Geometry: final body of the model. Coordinates: model frame, mm. A direction names the side the tool comes from. Round coordinates to 2 decimals unless told otherwise and drop trailing zeros. Loops run counter-clockwise (first coordinate to the right, second up) from the corner with the lowest first, then second, coordinate; pieces in that order, holes last. Notation, with made-up numbers: (10.5, 9.25) - (46.5, 9.25) arc R31 ccw to (46.5, 39.25) - close; hole circle Ø4 at (-21.75, 4.5). An arc over 180 degrees is marked (long way). Answer as a JSON object with one key per item and string values. Group by question number.
Item 1: Section D-D (z = 42.5). Return the cut outline in (x, y), plus the area to 3 significant figures.
Item 2: First-contact query: pin 1 (2 mm diameter, centred on y = 15, z = 30.5, fed in from -X); pin 2 (4 mm diameter, centred on x = 44.5, z = -7, fed in from +Y); pin 3 (4 mm diameter, centred on x = 51.16, z = 29.39, fed in from -Y). Flat tips, straight axial feed; report the tip coordinate or a pass-through.
Item 3: Section C-C (x = 40). Return the cut outline in (y, z), plus the area to 3 significant figures.
Item 4: Section B-B (y = 14). Return the cut outline in (x, z).
Item 5: Reachability of faces 4 (the face through (-49.787, 24.294, -11.056)), 5 (the face through (-56, 41, 0)), 6 (the face through (50.249, 43.028, 28.195)) from +Z, -Z, +X, -X, +Y, -Y: full face, straight path, thin tool, end or side. Return the list, or none.
Item 6: Section A-A (z = 0). Return the cut outline in (x, y).
Item 7: Line query: line 1 (Z direction, x = 1.5, y = 22.5); line 2 (X direction, y = 1, z = 0); line 3 (X direction, y = 17.5, z = 0). Output: solid intervals per line, ascending.
Item 8: Draft query along Z for faces 1 (the face through (62.464, 42.972, -8.201)), 2 (the face through (-11, 0, -1)), 3 (the face through (-4.88, 1.48, 1.08)). Return one class per face: released by +Z, released by -Z, zero draft, split by the parting line, or undercut.
```python
from build123d import *

# Parameters (mm, degrees)
SKETCH1_R           = 55
BOSS_EXTRUDE1_DEPTH = 41
SKETCH2_R           = 63
BOSS_EXTRUDE2_DEPTH = 4
SKETCH3_R           = 51
CUT_EXTRUDE3_DEPTH  = 42
SKETCH4_R           = 5
CUT_EXTRUDE4_DEPTH  = 3
SKETCH5_R           = 1.5
CUT_EXTRUDE5_DEPTH  = 4


with BuildPart() as part:
    # Sketch1 → Boss-Extrude1 (new body)
    with BuildSketch(Plane(origin=(0, 0, 0), x_dir=(1, 0, 0), z_dir=(0, 1, 0))):
        with Locations(Location((0, 0, 0), (0, 0, 270))):
            Circle(SKETCH1_R)
    extrude(amount=BOSS_EXTRUDE1_DEPTH)

    # Sketch2 → Boss-Extrude2 (add)
    with BuildSketch(Plane(origin=(0, 41, 0), x_dir=(1, 0, 0), z_dir=(0, 1, 0))):
        with Locations(Location((0, 0, 0), (0, 0, 270))):
            Circle(SKETCH2_R)
    extrude(amount=BOSS_EXTRUDE2_DEPTH)

    # Sketch3 → Cut-Extrude3 (cut)
    with BuildSketch(Plane(origin=(0, 45, 0), x_dir=(1, 0, 0), z_dir=(0, 1, 0))):
        with Locations(Location((0, 0, 0), (0, 0, 270))):
            Circle(SKETCH3_R)
    extrude(amount=-CUT_EXTRUDE3_DEPTH, mode=Mode.SUBTRACT)

    # Sketch4 → Cut-Extrude4 (cut)
    with BuildSketch(Plane.XZ):
        with Locations(Location((0, 0, 0), (0, 0, 270))):
            Circle(SKETCH4_R)
    extrude(amount=-CUT_EXTRUDE4_DEPTH, mode=Mode.SUBTRACT)

    # Sketch5 → Cut-Extrude5 (cut)
    with BuildSketch(Plane(origin=(0, 45, 0), x_dir=(1, 0, 0), z_dir=(0, 1, 0))):
        with Locations(Location((-0.350950897, 58.998956207, 0), (0, 0, 270))):
            Circle(SKETCH5_R)
        with Locations(Location((-51.138331167, -29.42568751, 0), (0, 0, 270))):
            Circle(SKETCH5_R)
        with Locations(Location((51.161668833, -29.385092176, 0), (0, 0, 270))):
            Circle(SKETCH5_R)
    extrude(amount=-CUT_EXTRUDE5_DEPTH, mode=Mode.SUBTRACT)


solid = part.part
```
Values:
{
 "1": {"outline": "(-46.51, 41) - (-34.91, 41) - (-34.91, 0) - (34.91, 0) - (34.91, 41) - (46.51, 41) - (46.51, 45) - (28.19, 45) - (28.19, 3) - (-28.19, 3) - (-28.19, 45) - (-46.51, 45) - close", "area": "867 mm^2"},
 "2": {"pin 1": "stops at x = -46.42", "pin 2": "stops at y = 3", "pin 3": "stops at y = 41"},
 "3": {"outline": "(0, -37.75) - (41, -37.75) - (41, -48.67) - (45, -48.67) - (45, -31.64) - (3, -31.64) - (3, 31.64) - (45, 31.64) - (45, 48.67) - (41, 48.67) - (41, 37.75) - (0, 37.75) - close", "area": "827 mm^2"},
 "4": {"outline": "circle Ø110 at (0, 0); hole circle Ø102 at (0, 0)"},
 "5": {"face 4": "+Y", "face 5": "-Y", "face 6": "+Y, -Y"},
 "6": {"outline": "(-63, 41) - (-55, 41) - (-55, 0) - (-5, 0) - (-5, 3) - (-51, 3) - (-51, 45) - (-63, 45) - close; (5, 0) - (55, 0) - (55, 41) - (63, 41) - (63, 45) - (51, 45) - (51, 3) - (5, 3) - close"},
 "7": {"line 1": "z = -54.98 to -50.98, 50.98 to 54.98", "line 2": "x = -55 to -5, 5 to 55", "line 3": "x = -55 to -51, 51 to 55"},
 "8": {"face 1": "split by the parting line", "face 2": "zero draft", "face 3": "undercut"}
}
